Could you check a few things on this model? Use its own coordinates, in mm. Round coordinates to 2 decimals unless told otherwise and drop trailing zeros. Loops run counter-clockwise (first coordinate to the right, second up) from the corner with the lowest first, then second, coordinate; pieces in that order, holes last. Notation, with made-up numbers: (-14, 6) -> (14, 6) arc R22 ccw to (14, 12) -> close; hole circle Ø10 at (89, 37). An arc over 180 degrees is marked (long way). Put each result on its own line as item: value. Start each with the question number.
1. Imagine slicing it at C-C, the plane x = -29. Please give me the cut outline in (y, z), and give its area (3 significant figures).
2. Imagine slicing it at B-B, the plane z = 14.5. Please give me the cut outline in (x, y).
3. I need wall thicknesses on line 1 (X direction, y = 9, z = 0); line 2 (Y direction, x = 0, z = -2.5); line 3 (X direction, y = 57.5, z = 17.5). Which ranges of each line are inside material? Lowest first, please. Write a range as [from, to].
4. I'm going to push flat-ended pins straight in: P1, Ø12, axis at y = 84, z = 19, coming from the -X side; P2, Ø2.5, axis at x = 1, z = -1.5, coming from the -Y side; P3, Ø3, axis at y = 90.5, z = -0.5, coming from the +X side; P4, Ø8, axis at y = 88, z = 26.5, coming from the -X side. Where does each tip first touch, or does it pass through?
5. Imagine slicing it at A-A, the plane y = 86.5. Please give me the cut outline in (x, z), and give its area (3 significant figures).
```python
from build123d import *

# Parameters (mm, degrees)
PRISMA_HEXAGONAL_DEPTH     = 120
CROQUIS_AGUJEROS_MONTAJE_R = 4
AGUJERO_INSERTO_M6_DEPTH   = 14


with BuildPart() as part:
    # Croquis_hexagono → Prisma_hexagonal (new body)
    with BuildSketch(Plane(origin=(0, 0, 0), x_dir=(1, 0, 0), z_dir=(0, 1, 0))):
        Polygon((40, 0), (20, 34.641016151), (-20, 34.641016151), (-40, 0), (-20, -34.641016151), (20, -34.641016151), align=None)
    extrude(amount=PRISMA_HEXAGONAL_DEPTH)

    # Croquis_agujeros_montaje → Agujero_inserto_M6 (cut)
    with BuildSketch(Plane(origin=(0, 0, 0), x_dir=(1, 0, 0), z_dir=(0, 1, 0))):
        with Locations(Location((0, 0, 0), (0, 0, 270))):
            Circle(CROQUIS_AGUJEROS_MONTAJE_R)
    extrude(amount=AGUJERO_INSERTO_M6_DEPTH, mode=Mode.SUBTRACT)


solid = part.part
```
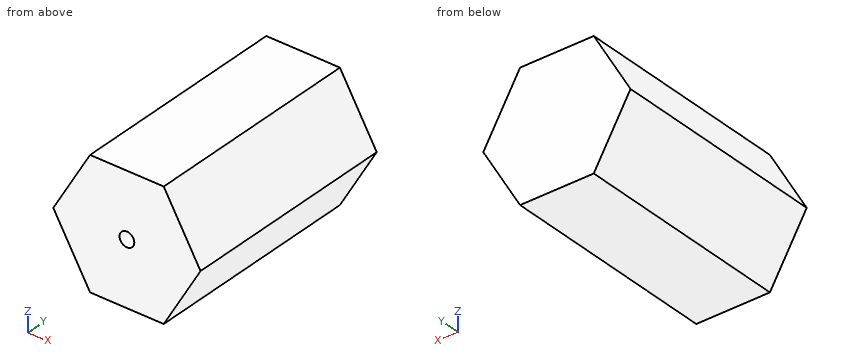
Entries:
1. outline: (0, -19.05) -> (120, -19.05) -> (120, 19.05) -> (0, 19.05) -> close
1. area: 4,570 mm^2
2. outline: (-31.63, 0) -> (31.63, 0) -> (31.63, 120) -> (-31.63, 120) -> close
3. line 1: [-40, -4], [4, 40]
3. line 2: [14, 120]
3. line 3: [-29.9, 29.9]
4. P1: x = -32.49
4. P2: y = 14
4. P3: x = 40
4. P4: x = -27.01
5. outline: (-40, 0) -> (-20, -34.64) -> (20, -34.64) -> (40, 0) -> (20, 34.64) -> (-20, 34.64) -> close
5. area: 4,160 mm^2
